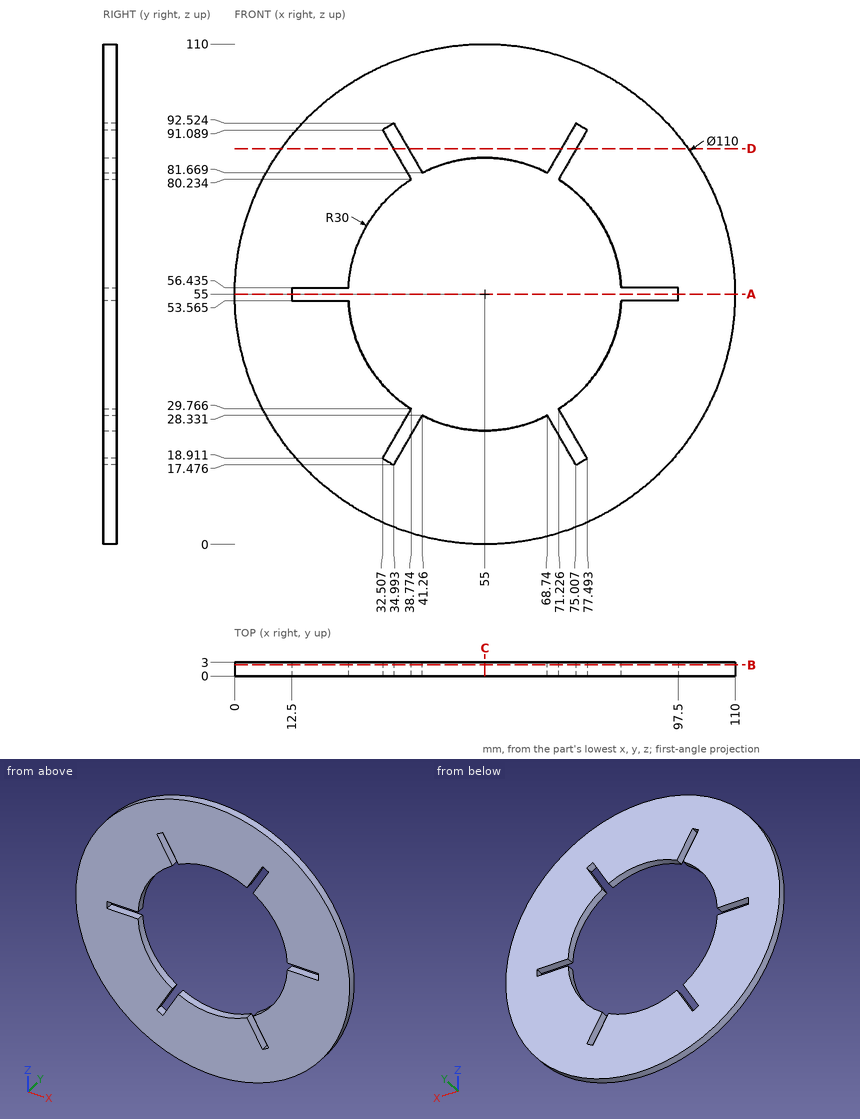
Print and shaded views of the part. All mm, measured from the part's lowest x, y and z. Give positions to 0.01 mm unless a question says otherwise; leave off trailing zeros. Loops run counter-clockwise (first coordinate to the right, second up) from the corner with the lowest first, then second, coordinate; pieces in that order, holes last. Notation, with made-up numbers: (71, -11.5) -> (123, -11.5) arc R25 ccw to (123, 0.5) -> close; hole circle Ø6 at (35.5, -38). An arc over 180 degrees is marked (long way). One line per question, with ' | ' between items. Start each with the question number.
1) Cut at B-B (y = 2.45). Give the cut face in (x, z) (1 decimal), plus the area to 3 significant figures.
2) Cut at A-A (z = 55). Give the cut face in (x, y).
3) Cut at D-D (z = 87). Give the cut face in (x, y).
4) Pin check, flat tips, straight feed: pin 1 (1.4 mm diameter, centred on y = 1, z = 55.5, fed in from -X); pin 2 (1.5 mm diameter, centred on y = 1.5, z = 56.5, fed in from +X) (1 decimal); pin 3 (1.5 mm diameter, centred on x = 16, y = 1.5, fed in from -Z). Stop position of each tip, or through.
5) Cut at C-C (x = 55). Give the cut face in (y, z), plus the area to 3 significant figures.
6) Probe L1, parallel to X at y = 2, z = 54; L2, parallel to X at y = 1.5, z = 19 (1 decimal); L3, parallel to X at y = 2.35, z = 87. List the from-to ranges inside material, lowest first.
Return value:
1) outline: circle Ø110 at (55, 55); hole (12.5, 53.6) -> (25, 53.6) arc R30 ccw to (38.8, 29.8) -> (32.5, 18.9) -> (35, 17.5) -> (41.3, 28.3) arc R30 ccw to (68.7, 28.3) -> (75, 17.5) -> (77.5, 18.9) -> (71.2, 29.8) arc R30 ccw to (85, 53.6) -> (97.5, 53.6) -> (97.5, 56.4) -> (85, 56.4) arc R30 ccw to (71.2, 80.2) -> (77.5, 91.1) -> (75, 92.5) -> (68.7, 81.7) arc R30 ccw to (41.3, 81.7) -> (35, 92.5) -> (32.5, 91.1) -> (38.8, 80.2) arc R30 ccw to (25, 56.4) -> (12.5, 56.4) -> close | area: 6,460 mm^2
2) outline: (0, 0) -> (12.5, 0) -> (12.5, 3) -> (0, 3) -> close; (97.5, 0) -> (110, 0) -> (110, 3) -> (97.5, 3) -> close
3) outline: (10.27, 0) -> (34.87, 0) -> (34.87, 3) -> (10.27, 3) -> close; (38.18, 0) -> (71.82, 0) -> (71.82, 3) -> (38.18, 3) -> close; (75.13, 0) -> (99.73, 0) -> (99.73, 3) -> (75.13, 3) -> close
4) pin 1: x = 0 | pin 2: x = 110 | pin 3: z = 15.48
5) outline: (0, 0) -> (3, 0) -> (3, 25) -> (0, 25) -> close; (0, 85) -> (3, 85) -> (3, 110) -> (0, 110) -> close | area: 150 mm^2
6) L1: 0.01 to 12.5, 97.5 to 109.99 | L2: 13.4 to 32.6, 35.9 to 74.1, 77.4 to 96.6 | L3: 10.27 to 34.87, 38.18 to 71.82, 75.13 to 99.73
